Geometry: final body of the model. Coordinates: model frame, mm. A direction names the side the tool comes from. Coordinates: 2 decimals unless noted, no trailing zeros. Order: outer loops, then holes, each group sorted by start corner. A loop starts at its lowest first (then second) coordinate and runs counter-clockwise, first axis right, second up. Notation, with made-up numbers: M -12.5,-20.75 L 19.5,-20.75 A15 cw 19.5,-9.75 Z; hole C 61.25,72 d7. An arc over 180 degrees is marked long. Write item = value, one per line.
Autodesk Inventor part; units mm, degrees
ref_plane "YZ Plane" through (0, 0, 0) normal (1, 0, 0) x (0, 1, 0)
ref_plane "XZ Plane" through (0, 0, 0) normal (0, 1, 0) x (-1, 0, 0)
ref_plane "XY Plane" through (0, 0, 0) normal (0, 0, 1) x (1, 0, 0)
sketch "Sketch1" plane through (0, 0, 0) normal (1, 0, 0) x (0, 1, 0)
  circle A0 centre (0, 0) radius 86.5188
  circle A1 centre (0, 63.5) radius 4.7625
  circle A2 centre (-44.9013, 44.9013) radius 4.7625
  circle A3 centre (-63.5, 0) radius 4.7625
  circle A4 centre (-44.9013, -44.9013) radius 4.7625
  circle A5 centre (0, -63.5) radius 4.7625
  circle A6 centre (44.9013, -44.9013) radius 4.7625
  circle A7 centre (63.5, 0) radius 4.7625
  circle A8 centre (44.9013, 44.9013) radius 4.7625
  line L0 (-31.75, 9.525) -> (31.75, 9.525)
  line L1 (31.75, 9.525) -> (31.75, -9.525)
  line L2 (31.75, -9.525) -> (-31.75, -9.525)
  line L3 (-31.75, -9.525) -> (-31.75, 9.525)
  circle A9 centre (0, 15.875) radius 1.5875
  circle A10 centre (-25.4, 15.875) radius 1.5875
  circle A11 centre (25.4, 15.875) radius 1.5875
  circle A12 centre (0, -15.875) radius 1.5875
  circle A13 centre (-25.4, -15.875) radius 1.5875
  circle A14 centre (25.4, -15.875) radius 1.5875
  circle A15 centre (-38.1, 0) radius 1.5875
  circle A16 centre (38.1, 0) radius 1.5875
  point P0 (0, 9.525)
  point P1 (-31.75, 0)
  dimension "d0" = 173.0375
  dimension "d3" = 360
  dimension "d5" = 9.525
  dimension "d6" = 63.5
  dimension "d7" = 63.5
  dimension "d8" = 19.05
  dimension "d9" = 3.175
  dimension "d10" = 15.875
  dimension "d13" = 25.4
  dimension "d20" = 25.4
  dimension "d27" = 31.75
  dimension "d32" = 38.1
  dimension "d33" = 3.175
  dimension "d36" = 76.2
extrude "Extrusion1" add sketch "Sketch1" along normal blind 76.2
hole "Hole1" at (76.2, 0, 0) direction (-1, 0, 0) diameter 171.45 depth 75.4062
properties part number "top cap"
1) Pin query (flat end, axial travel): pin 1 (1.9 mm diameter, centred on y = 25.4, z = 15.875, fed in from +X); pin 2 (15 mm diameter, centred on y = -44.9, z = -44.9, fed in from +X); pin 3 (0.6 mm diameter, centred on x = 0, y = 2, fed in from +Z); pin 4 (1.5 mm diameter, centred on x = 56.5, y = -20.5, fed in from +Z). Return the tip coordinate at first contact, or that it passes through.
Numbers:
pin_1 = through
pin_2 = 0.79
pin_3 = 86.5
pin_4 = 84.23
2) Section C-C, the plane x = 23.5. Return loops of the section in (y, z) (3 decimals).
Numbers:
outline = C 0,0 d173.038; hole C 0,0 d171.45
3) Line query: L1, parallel to Y at x = 5, z = -2; L2, parallel to Z at x = 0.35, y = -25.4 (1 decimal); L3, parallel to Z at x = 0.3, y = -63.5. Output: solid intervals per line, ascending.
Numbers:
L1 = -86.5 to -85.7, 85.7 to 86.5
L2 = -82.7 to -17.5, -14.3 to -9.5, 9.5 to 14.3, 17.5 to 82.7
L3 = -58.76 to -4.76, 4.76 to 58.76
4) Section A-A, the plane y = -63. Return loops of the section in (x, z), and give its area (3 significant figures).
Numbers:
outline = M 0,-59.3 L 76.2,-59.3 L 76.2,-58.14 L 0.79,-58.14 L 0.79,-4.74 L 0,-4.74 Z; M 0,4.74 L 0.79,4.74 L 0.79,58.14 L 76.2,58.14 L 76.2,59.3 L 0,59.3 Z
area = 262 mm²
5) Section D-D, the plane y = 63.5. Return loops of the section in (x, z), and give its area (3 significant figures).
Numbers:
outline = M 0,-58.76 L 76.2,-58.76 L 76.2,-57.59 L 0.79,-57.59 L 0.79,-4.76 L 0,-4.76 Z; M 0,4.76 L 0.79,4.76 L 0.79,57.59 L 76.2,57.59 L 76.2,58.76 L 0,58.76 Z
area = 263 mm²
6) Section B-B, the plane z = 26. Return loops of the section in (x, y), and give its area (3 significant figures).
Numbers:
outline = M 0,-82.52 L 76.2,-82.52 L 76.2,-81.69 L 0.79,-81.69 L 0.79,81.69 L 76.2,81.69 L 76.2,82.52 L 0,82.52 Z
area = 257 mm²
7) Set-up query: faces 5 (the face through (0.794, -1, -18)), 6 (the face through (0.39, -0.62, 58.78)). Return all of +Z, -Z, +X, -X, +Y, -Y with unobstructed straight access to the full face (end or side cutting, diameter ignored); none if empty.
Numbers:
face_5 = +X
face_6 = +X, -X
8) Mould query, pull axis Y, two halves, no side actions, for faces 1 (the face through (0.391, 49.444, -46.332)), 2 (the face through (76.2, -84, 20)), 3 (the face through (37.567, 82.524, -25.988)), 4 (the face through (0.391, 47.462, 40.886)). Classes: pulls with the +Y half, pulls with the -Y half, needs draft (parallel to the pull), parting line crosses it, or undercut.
Numbers:
face_1 = undercut
face_2 = needs draft
face_3 = parting line crosses it
face_4 = undercut
